Here's how the part is built. I have some questions about the finished solid (model axes, mm). Coordinates: 2 decimals unless noted, no trailing zeros. Write each loop counter-clockwise with the first axis right and the second up, starting at its lowest first coordinate (ties: lowest second). Pieces come first, ordered by that corner, then holes.
(1) Imagine slicing it at A-A, the plane z = 0.35. List the corners of the cut face in (x, y) for me.
(2) Please list where these lines run through material, in increasing order: probe 1 along Y at (x, z) = (22.5, 0.9); probe 2 along Y at (x, z) = (-54.5, 1.5); probe 3 along X at (y, z) = (-3.5, 1.7).
(3) Imagine slicing it at D-D, the plane x = 46.5. List the corners of the cut face in (y, z) for me, plus the area to 3 significant figures.
(4) For pin 1 Ø12 at (x, y) = (-0.5, 26.5) entering from -Z, with a flat end and sliding along its axis, tell me the tip position at first contact or that it passes through.
(5) Imagine slicing it at C-C, the plane y = 0. List the corners of the cut face in (x, z) for me.
(6) Imagine slicing it at B-B, the plane x = -54.5. List the corners of the cut face in (y, z) for me, plus the area to 3 significant figures.
(7) Thinking about a two-plate mould opening in Y: for faces 1 (the cylindrical face through (24.95, -1.01, 1.01)), 2 (the flat face through (-1, 0, 2)), which applies, released by +Y, released by -Y, zero draft, split by the parting line, or undercut?
```python
from build123d import *

# Parameters (mm, degrees)
SKETCH1_W           = 145
SKETCH1_H           = 68
BOSS_EXTRUDE1_DEPTH = 2
SKETCH2_R           = 8
SKETCH2_R_2         = 2.65
CUT_EXTRUDE1_DEPTH  = 81.101498113


with BuildPart() as part:
    # Sketch1 → Boss-Extrude1 (new body)
    with BuildSketch(Plane.XY):
        Rectangle(SKETCH1_W, SKETCH1_H)
    extrude(amount=BOSS_EXTRUDE1_DEPTH)

    # Sketch2 → Cut-Extrude1 (cut, through all)
    with BuildSketch(Plane.XY.offset(2)):
        with Locations((-54.5, 0)):
            Circle(SKETCH2_R)
        with Locations((22.5, 0)):
            Circle(SKETCH2_R_2)
        with BuildLine():
            Line((61.5, -13), (41.9, -13))
            ThreePointArc((41.9, -13), (41.192893219, -12.707106781), (40.9, -12))
            Line((40.9, -12), (40.9, 12))
            ThreePointArc((40.9, 12), (41.192893219, 12.707106781), (41.9, 13))
            Line((41.9, 13), (61.5, 13))
            ThreePointArc((61.5, 13), (62.207106781, 12.707106781), (62.5, 12))
            Line((62.5, 12), (62.5, -12))
            ThreePointArc((62.5, -12), (62.207106781, -12.707106781), (61.5, -13))
        make_face()
    extrude(amount=-CUT_EXTRUDE1_DEPTH, mode=Mode.SUBTRACT)


solid = part.part
```
Recorded:
1. outline: (-72.5, -34) - (72.5, -34) - (72.5, 34) - (-72.5, 34) - close; hole circle Ø16 at (-54.5, 0); hole circle Ø5.3 at (22.5, 0); hole (40.9, -12) arc R1 ccw to (41.9, -13) - (61.5, -13) arc R1 ccw to (62.5, -12) - (62.5, 12) arc R1 ccw to (61.5, 13) - (41.9, 13) arc R1 ccw to (40.9, 12) - close
2. probe 1: y = -34 to -2.65, 2.65 to 34
2. probe 2: y = -34 to -8, 8 to 34
2. probe 3: x = -72.5 to -61.69, -47.31 to 40.9, 62.5 to 72.5
3. outline: (-34, 0) - (-13, 0) - (-13, 2) - (-34, 2) - close; (13, 0) - (34, 0) - (34, 2) - (13, 2) - close
3. area: 84.0 mm2
4. pin 1: stops at z = 0
5. outline: (-72.5, 0) - (-62.5, 0) - (-62.5, 2) - (-72.5, 2) - close; (-46.5, 0) - (19.85, 0) - (19.85, 2) - (-46.5, 2) - close; (25.15, 0) - (40.9, 0) - (40.9, 2) - (25.15, 2) - close; (62.5, 0) - (72.5, 0) - (72.5, 2) - (62.5, 2) - close
6. outline: (-34, 0) - (-8, 0) - (-8, 2) - (-34, 2) - close; (8, 0) - (34, 0) - (34, 2) - (8, 2) - close
6. area: 104 mm2
7. face 1: undercut
7. face 2: zero draft
